from build123d import *

# Parameters (mm, degrees)
F0_R     = 1.7272
F0_R_2   = 3.96875
F0_R_3   = 17.145
F0_R_4   = 11.1125
F0_R_5   = 6.5875027
F1_DEPTH = 3.175
F3_DEPTH = 3.175
F4_COUNT = 6
F4_ANGLE = 300
F5_R     = 4.7625


with BuildPart() as f1:
    # F0 (on Top) → F1 (new body)
    with BuildSketch(Plane.XY):
        with BuildLine():
            Line((-303.6125627, 32.54375), (-346.1094200534, 21.5120031198))
            ThreePointArc((-346.1094200534, 21.5120031198), (-362.7501254, 0), (-346.1094200534, -21.5120031198))
            Line((-346.1094200534, -21.5120031198), (-303.6125627, -32.54375))
            Line((-303.6125627, -32.54375), (-297.2625627, -32.54375))
            Line((-297.2625627, -32.54375), (-297.2625627, -29.36875))
            Line((-297.2625627, -29.36875), (-43.2625627, -29.36875))
            Line((-43.2625627, -29.36875), (-43.2625627, -32.54375))
            Line((-43.2625627, -32.54375), (-36.9125627, -32.54375))
            Line((-36.9125627, -32.54375), (1.6456052558, -22.5344463586))
            Line((1.6456052558, -22.5344463586), (24.6620081426, -45.5508492454))
            ThreePointArc((24.6620081426, -45.5508492454), (26.2070743414, -46.5832294736), (28.029604188, -46.9457532))
            Line((28.029604188, -46.9457532), (69.9924832184, -46.9457532))
            Line((69.9924832184, -46.9457532), (69.9924832184, 46.9457532))
            Line((69.9924832184, 46.9457532), (28.029604188, 46.9457532))
            ThreePointArc((28.029604188, 46.9457532), (26.2070743414, 46.5832294736), (24.6620081426, 45.5508492454))
            Line((24.6620081426, 45.5508492454), (1.6456052558, 22.5344463586))
            Line((1.6456052558, 22.5344463586), (-36.9125627, 32.54375))
            Line((-36.9125627, 32.54375), (-43.2625627, 32.54375))
            Line((-43.2625627, 32.54375), (-43.2625627, 29.36875))
            Line((-43.2625627, 29.36875), (-297.2625627, 29.36875))
            Line((-297.2625627, 29.36875), (-297.2625627, 32.54375))
            Line((-297.2625627, 32.54375), (-303.6125627, 32.54375))
        make_face()
        with Locations((-282.9750627, -24.60625)):
            Circle(F0_R, mode=Mode.SUBTRACT)
        with Locations((-352.3117115589, -11.7865861589)):
            Circle(F0_R, mode=Mode.SUBTRACT)
        with Locations((-328.7385392411, -11.7865861589)):
            Circle(F0_R_2, mode=Mode.SUBTRACT)
        with Locations((-57.5500627, -24.60625)):
            Circle(F0_R, mode=Mode.SUBTRACT)
        with Locations((-11.7865861589, -11.7865861589)):
            Circle(F0_R_2, mode=Mode.SUBTRACT)
        with Locations((11.7865861589, -11.7865861589)):
            Circle(F0_R, mode=Mode.SUBTRACT)
        with Locations((46.6297937032, -18.95475)):
            Circle(F0_R_3, mode=Mode.SUBTRACT)
        with Locations((-340.5251254, 0)):
            Circle(F0_R_4, mode=Mode.SUBTRACT)
        with Locations((-289.7251254, 0)):
            Circle(F0_R, mode=Mode.SUBTRACT)
        with Locations((-352.3117115589, 11.7865861589)):
            Circle(F0_R_2, mode=Mode.SUBTRACT)
        with Locations((-328.7385392411, 11.7865861589)):
            Circle(F0_R, mode=Mode.SUBTRACT)
        with Locations((-282.9750627, 24.60625)):
            Circle(F0_R, mode=Mode.SUBTRACT)
        with Locations((-50.8, 0)):
            Circle(F0_R, mode=Mode.SUBTRACT)
        Circle(F0_R_4, mode=Mode.SUBTRACT)
        with Locations((28.029604188, 5.55625)):
            Circle(F0_R, mode=Mode.SUBTRACT)
        with Locations((65.2299832184, 5.55625)):
            Circle(F0_R, mode=Mode.SUBTRACT)
        with Locations((-11.7865861589, 11.7865861589)):
            Circle(F0_R, mode=Mode.SUBTRACT)
        with Locations((11.7865861589, 11.7865861589)):
            Circle(F0_R_2, mode=Mode.SUBTRACT)
        with Locations((-57.5500627, 24.60625)):
            Circle(F0_R, mode=Mode.SUBTRACT)
        with Locations((46.6297937032, 26.32075)):
            Circle(F0_R_5, mode=Mode.SUBTRACT)
        with Locations((28.029604188, 42.1832532)):
            Circle(F0_R, mode=Mode.SUBTRACT)
        with Locations((65.2299832184, 42.1832532)):
            Circle(F0_R, mode=Mode.SUBTRACT)
    extrude(amount=F1_DEPTH)

    # F2 (on face) → F3 (cut, through all)
    with BuildSketch(Plane(origin=(0, 0, 0), x_dir=(1, 0, 0), z_dir=(0, 0, -1))):
        with BuildLine():
            ThreePointArc((-348.3828495059, -7.8577241059), (-350.1488326996, -5.55625), (-351.2589761446, -2.8761266387))
            Line((-351.2589761446, -2.8761266387), (-352.0256797693, -3.0815642558))
            ThreePointArc((-352.0256797693, -3.0815642558), (-350.8362403638, -5.953125), (-348.9441155135, -8.4189901135))
            Line((-348.9441155135, -8.4189901135), (-348.3828495059, -7.8577241059))
        make_face()
    f3 = extrude(amount=-F3_DEPTH, mode=Mode.SUBTRACT)

    # F4: F3 ×6 about axis
    f4_axis = Axis((-340.5251254, 0, 0), (0, 0, -1))
    for i in range(1, F4_COUNT):
        add(f3.rotate(f4_axis, i * F4_ANGLE / (F4_COUNT - 1)), mode=Mode.SUBTRACT)

    # F5
    f5_edges = [f1.edges().sort_by_distance(p)[0] for p in [
        (69.992483, 46.945753, 1.5875),
        (69.992483, -46.945753, 1.5875),
    ]]
    fillet(f5_edges, radius=F5_R)


solid = f1.part
Build history of the part. All positions in model axes, mm. A direction names the side the tool comes from. Round coordinates to 2 decimals unless told otherwise and drop trailing zeros. Write each loop counter-clockwise with the first axis right and the second up, starting at its lowest first coordinate (ties: lowest second). Pieces come first, ordered by that corner, then holes. Notation, with made-up numbers: M 47,-32.75 L 86,-32.75 A19 cw 86,0.25 Z; hole C -33,51 d8. An arc over 180 degrees is marked long. Use CSV: the item, a comma, the result in double quotes.
1. Tool access for faces 5 (the face through (13.31, 34.2, 1.57)), 6 (the face through (-325.16, -26.95, 1.57)), 7 (the face through (-17.9, -27.61, 1.57)): list every direction of +Z, -Z, +X, -X, +Y, -Y with a clear straight run to the whole face (end or side of a thin tool).
Reply:
face 5,"+Z, -Z, +Y"
face 6,"+Z, -Z, -X, -Y"
face 7,"+Z, -Z, -Y"
2. Saw through at B-B (z = 1.7). State how many separate pieces and enclosed holes the cut face has, plus the area to 3 significant figures.
Reply:
separate pieces,"1"
enclosed holes,"22"
area,"24,300 mm²"
3. Flat gauge pins, fed straight in: pin 1 (1 mm diameter, centred on y = 4.5, z = 2.5, fed in from -X); pin 2 (3 mm diameter, centred on x = 11.79, y = -11.79, fed in from -Z); pin 3 (1 mm diameter, centred on x = -135.5, z = 0.5, fed in from +Y); pin 4 (1 mm diameter, centred on y = 6.5, z = 3, fed in from -X). Where does each tip first touch, or does it go through?
Reply:
pin 1,"stops at x = -362.39"
pin 2,"passes through"
pin 3,"stops at y = 29.37"
pin 4,"stops at x = -361.92"
4. Wall check: probe 1 along X at (y, z) = (7, 2.2); probe 2 along X at (y, z) = (6.5, 1.8); probe 3 along Y at (x, z) = (0, 2). Give the ranges that are in metal, low to high. Write a range as from..to.
Reply:
probe 1,"x = -361.62..-350.16, -330.89..-8.63, 8.63..27.08, 28.98..64.28, 66.18..69.99"
probe 2,"x = -361.78..-350.5, -330.55..-9.01, 9.01..26.58, 29.48..63.78, 66.68..69.99"
probe 3,"y = -22.96..-11.11, 11.11..22.96"
5. Saw through at A-A (x = -74). Give the cut face in (y, z) (3 decimals).
Reply:
outline,"M -29.369,0 L 29.369,0 L 29.369,3.175 L -29.369,3.175 Z"
6. Two-plate mould, pull along X, no slides. Class faces 1 (the face through (-149, 1, 0)), 2 (the face through (12.99, -33.88, 1.57)), 3 (the face through (-324.953, -10.594, 1.565)), 4 (the face through (-362.746, 0.41, 1.565)): +X half, -X half, draft (parallel to the pull), parting line (faces both ways), or undercut.
Reply:
face 1,"draft"
face 2,"undercut"
face 3,"undercut"
face 4,"-X half"
7. Saw through at C-C (x = -27). Give the cut face in (y, z) (3 decimals), plus the area to 3 significant figures.
Reply:
outline,"M -29.971,0 L 29.971,0 L 29.971,3.175 L -29.971,3.175 Z"
area,"190 mm²"
